Verification items for this drawing (mm, ordinates from the low corner). A direction names the side the tool comes from. Round coordinates to 2 decimals unless told otherwise and drop trailing zeros. Write each loop counter-clockwise with the first axis right and the second up, starting at its lowest first coordinate (ties: lowest second). Pieces come first, ordered by that corner, then holes. Notation, with made-up numbers: M -3,-21.5 L 34,-21.5 A5 cw 34,-17.5 Z; hole C 65.5,63 d2. An arc over 180 degrees is marked long. Write each question's results on one line, items separated by ' | '.
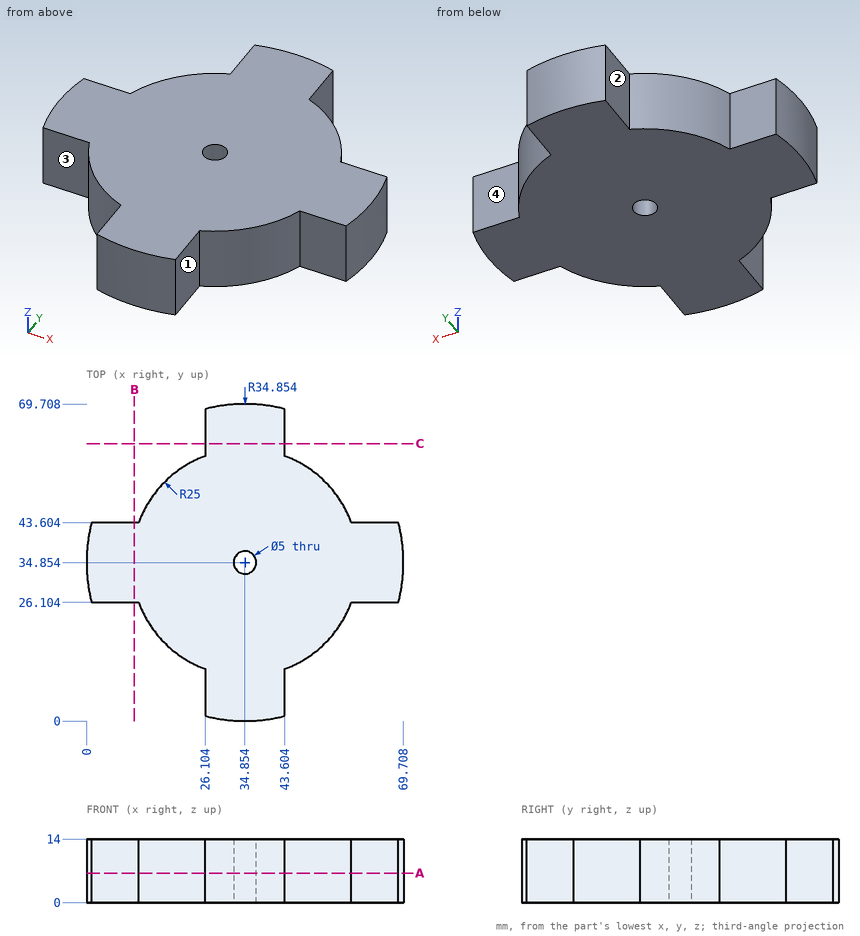
1) Access from +Z, -Z, +X, -X, +Y, -Y to the whole of each face (thin tool, end or side, straight path). Record for the marked faces 1, 2, 3 and 4.
Calculated:
face 1: +Z, -Z, +X, -Y | face 2: +Z, -Z, -X, +Y | face 3: +Z, -Z, -X, -Y | face 4: +Z, -Z, +X, +Y
2) Material ranges on line 1 (Y direction, x = 63.5, z = 10); line 2 (X direction, y = 51, z = 1.5), recorded low to high. Write a range as [from, to].
Calculated:
line 1: y = [26.1, 43.6] | line 2: x = [15.77, 53.94]
3) Sectioned sample at A-A, the plane z = 6.5. Record the cut outline in (x, y).
Calculated:
outline: M 1.12,26.1 L 11.44,26.1 A25 ccw 26.1,11.44 L 26.1,1.12 A34.85 ccw 43.6,1.12 L 43.6,11.44 A25 ccw 58.27,26.1 L 68.59,26.1 A34.85 ccw 68.59,43.6 L 58.27,43.6 A25 ccw 43.6,58.27 L 43.6,68.59 A34.85 ccw 26.1,68.59 L 26.1,58.27 A25 ccw 11.44,43.6 L 1.12,43.6 A34.85 ccw Z; hole C 34.85,34.85 d5
4) Depth check by flat-ended pin: P1, Ø3, axis at y = 8.5, z = 9.5, coming from the -X side; P2, Ø4, axis at x = 17.5, z = 2, coming from the +Y side; P3, Ø5, axis at y = 6.5, z = 7, coming from the +X side. Enter the tip coordinate at first touch or a pass-through.
Calculated:
P1: stops at x = 26.1 | P2: stops at y = 54.58 | P3: stops at x = 43.6
5) Sectioned sample at B-B, the plane x = 10.5. Record the cut outline in (y, z), and give its area (3 significant figures).
Calculated:
outline: M 26.1,0 L 43.6,0 L 43.6,14 L 26.1,14 Z | area: 245 mm²
